```python
from build123d import *

# Parameters (mm, degrees)
SKETCH1_W           = 230
SKETCH1_H           = 150
BOSS_EXTRUDE3_DEPTH = 10
SKETCH3_W           = 220.032470936
SKETCH3_H           = 140.023771478
CUT_EXTRUDE1_DEPTH  = 8
FILLET1_R           = 1
FILLET2_R           = 1
FILLET3_R           = 1
SKETCH6_R           = 5
CUT_EXTRUDE3_DEPTH  = 10


with BuildPart() as part:
    # Sketch1 → Boss-Extrude3 (new body)
    with BuildSketch(Plane(origin=(0, 0, 0), x_dir=(1, 0, 0), z_dir=(0, 1, 0))):
        with Locations((115, 75)):
            Rectangle(SKETCH1_W, SKETCH1_H)
    extrude(amount=BOSS_EXTRUDE3_DEPTH)

    # Sketch3 → Cut-Extrude1 (cut)
    with BuildSketch(Plane(origin=(0, 10, 0), x_dir=(1, 0, 0), z_dir=(0, 1, 0))):
        with Locations((115, 75)):
            Rectangle(SKETCH3_W, SKETCH3_H)
    extrude(amount=-CUT_EXTRUDE1_DEPTH, mode=Mode.SUBTRACT)

    # Fillet1
    fillet1_edges = [part.edges().sort_by_distance(p)[0] for p in [
        (0, 5, 0),
    ]]
    fillet(fillet1_edges, radius=FILLET1_R)

    # Fillet2
    fillet2_edges = [part.edges().sort_by_distance(p)[0] for p in [
        (0, 5, -150),
        (230, 5, -150),
        (230, 5, 0),
    ]]
    fillet(fillet2_edges, radius=FILLET2_R)

    # Fillet3
    fillet3_edges = [part.edges().sort_by_distance(p)[0] for p in [
        (115, 0, 0),
        (0.292893219, 0, -0.292893219),
        (0, 0, -75),
        (115, 0, -150),
        (230, 0, -75),
        (229.707106781, 0, -149.707106781),
        (229.707106781, 0, -0.292893219),
        (0.292893219, 0, -149.707106781),
    ]]
    fillet(fillet3_edges, radius=FILLET3_R)

    # Sketch6 → Cut-Extrude3 (cut)
    with BuildSketch(Plane.XZ):
        with Locations((144.826508181, -48.408466726)):
            Circle(SKETCH6_R)
        with Locations((178.556568371, -48.408466726)):
            Circle(SKETCH6_R)
        with Locations((178.592552161, -75)):
            Circle(SKETCH6_R)
        with Locations((144.862491971, -75)):
            Circle(SKETCH6_R)
        with Locations((144.862491971, -102.290057641)):
            Circle(SKETCH6_R)
        with Locations((178.592552161, -102.290057641)):
            Circle(SKETCH6_R)
        with Locations((212.322612351, -75)):
            Circle(SKETCH6_R)
    extrude(amount=-CUT_EXTRUDE3_DEPTH, mode=Mode.SUBTRACT)


solid = part.part
```
Build history of the part. All positions in model axes, mm. A direction names the side the tool comes from. Round coordinates to 2 decimals unless told otherwise and drop trailing zeros. Write each loop counter-clockwise with the first axis right and the second up, starting at its lowest first coordinate (ties: lowest second). Pieces come first, ordered by that corner, then holes. Notation, with made-up numbers: (-4, -7.75) - (44, -7.75) arc R11 cw to (44, 3.25) - close; hole circle Ø5 at (78, 35). An arc over 180 degrees is marked (long way). Write each question's results on one line, items separated by ' | '. Start each with the question number.
Item 1: Drop flat-ended pins along their axis: P1, Ø9, axis at x = 178.59, z = -75, coming from the +Y side; P2, Ø5, axis at x = 179.5, z = -19.5, coming from the +Y side. Give the stop position or say it passes through.
Item 2: Saw through at D-D (x = 160). Write the cut outline in (y, z).
Item 3: Saw through at B-B (y = 4). Write the cut outline in (x, z), and give its area (3 significant figures).
Item 4: Saw through at A-A (z = -46). Write the cut outline in (x, y), and give its area (3 significant figures).
Item 5: Saw through at C-C (z = -75). Write the cut outline in (x, y).
Item 6: Wall check: L1, parallel to Z at x = 178.5, y = 1.75; L2, parallel to Z at x = 107.5, y = 2.75; L3, parallel to X at y = 7.75, z = -106.5. Give the ranges that are in metal, low to high. Write a range as [from, to].
Item 7: Which spindle directions (+Z, -Z, +X, -X, +Y, -Y) get a long thin tool onto all of the face, cutting with end or side? Do faces 4 (the face through (143.78, 0.99, -107.17)), 5 (the face through (4.984, 6, -74)). Say none if no direction does.
Item 8: Mould opens along X. For faces 1 (the face through (0, 5, -74)), 2 (the face through (113, 5, -150)), 3 (the face through (208.355, 0.986, -78.042)) say: pulls with the +X half, pulls with the -X half, needs draft (parallel to the pull), parting line crosses it, or undercut.
Results are:
1) P1: passes through | P2: stops at y = 2
2) outline: (0, -149) arc R1 ccw to (1, -150) - (10, -150) - (10, -145.01) - (2, -145.01) - (2, -4.99) - (10, -4.99) - (10, 0) - (1, 0) arc R1 ccw to (0, -1) - close
3) outline: (0, -149) arc R1 ccw to (1, -150) - (229, -150) arc R1 ccw to (230, -149) - (230, -1) arc R1 ccw to (229, 0) - (1, 0) arc R1 ccw to (0, -1) - close; hole (4.98, -145.01) - (225.02, -145.01) - (225.02, -4.99) - (4.98, -4.99) - close | area: 3,690 mm²
4) outline: (0, 1) arc R1 ccw to (1, 0) - (140.44, 0) - (140.44, 2) - (4.98, 2) - (4.98, 10) - (0, 10) - close; (149.21, 0) - (174.17, 0) - (174.17, 2) - (149.21, 2) - close; (182.94, 0) - (229, 0) arc R1 ccw to (230, 1) - (230, 10) - (225.02, 10) - (225.02, 2) - (182.94, 2) - close | area: 504 mm²
5) outline: (0, 1) arc R1 ccw to (1, 0) - (139.86, 0) - (139.86, 2) - (4.98, 2) - (4.98, 10) - (0, 10) - close; (149.86, 0) - (173.59, 0) - (173.59, 2) - (149.86, 2) - close; (183.59, 0) - (207.32, 0) - (207.32, 2) - (183.59, 2) - close; (217.32, 0) - (229, 0) arc R1 ccw to (230, 1) - (230, 10) - (225.02, 10) - (225.02, 2) - (217.32, 2) - close
6) L1: z = [-150, -107.29], [-97.29, -80], [-70, -53.41], [-43.41, 0] | L2: z = [-150, -145.01], [-4.99, 0] | L3: x = [0, 4.98], [225.02, 230]
7) face 4: +Y, -Y | face 5: +Y
8) face 1: pulls with the -X half | face 2: needs draft | face 3: undercut
